```python
from build123d import *

# Parameters (mm, degrees)
BASE_FLANGE1_DEPTH      = 31.75
F_1_4_CLEARANCE_HOLE1_D = 6.7564
F_1_4_CLEARANCE_HOLE2_D = 6.7564
FILLET1_R               = 2.54


# Sheet-metal steps are written as plain solids
with BuildPart() as part:
    # Sketch1 → Base-Flange1 (new body)
    with BuildSketch(Plane(origin=(0, 0, 0), x_dir=(0, 0, -1), z_dir=(1, 0, 0))):
        with BuildLine():
            Line((-28.575, 0), (-3.9878, 0))
            ThreePointArc((-3.9878, 0), (-1.167999578, 1.167999578), (0, 3.9878))
            Line((0, 3.9878), (0, 50.8))
            Line((0, 50.8), (-1.9939, 50.8))
            Line((-1.9939, 50.8), (-1.9939, 3.9878))
            ThreePointArc((-1.9939, 3.9878), (-2.577899789, 2.577899789), (-3.9878, 1.9939))
            Line((-3.9878, 1.9939), (-28.575, 1.9939))
            Line((-28.575, 1.9939), (-28.575, 0))
        make_face()
    extrude(amount=BASE_FLANGE1_DEPTH)

    # 1/4 Clearance Hole1 (through all)
    with Locations(Plane.XY.offset(1.9939)):
        with Locations((15.875, 41.275)):
            Hole(F_1_4_CLEARANCE_HOLE1_D / 2)

    # 1/4 Clearance Hole2 (through all)
    with Locations(Plane(origin=(0, 1.9939, 0), x_dir=(1, 0, 0), z_dir=(0, 1, 0))):
        with Locations((15.875, -22.225)):
            Hole(F_1_4_CLEARANCE_HOLE2_D / 2)

    # Fillet1
    fillet1_edges = [part.edges().sort_by_distance(p)[0] for p in [
        (31.75, 0.99695, 28.575),
        (0, 0.99695, 28.575),
        (31.75, 50.8, 0.99695),
        (0, 50.8, 0.99695),
    ]]
    fillet(fillet1_edges, radius=FILLET1_R)


solid = part.part
```
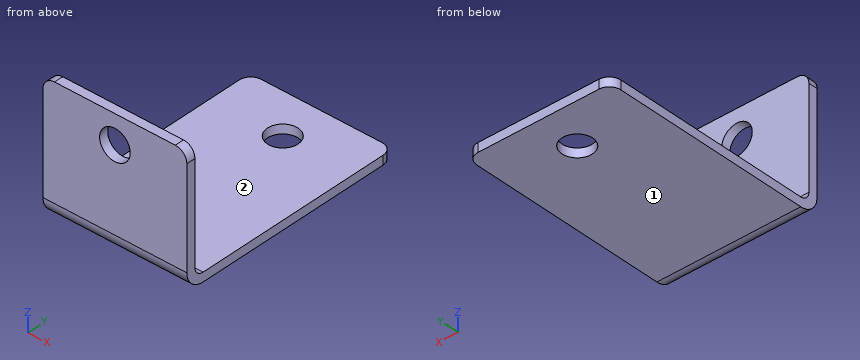
The listing builds one solid part. Answer for the finished solid, in the listing's coordinates (mm). Face numbers are marked on the shaded views. A direction names the side the tool comes from. Round coordinates to 2 decimals unless told otherwise and drop trailing zeros. Order: outer loops, then holes, each group sorted by start corner. A loop starts at its lowest first (then second) coordinate and runs counter-clockwise, first axis right, second up. Notation, with made-up numbers: (44, -6.75) -> (91, -6.75) arc R19 cw to (91, 18.25) -> close; hole circle Ø4 at (-34.5, 72.5). An arc over 180 degrees is marked (long way). Answer as CSV lines item,"result". Start each with the question number.
(1) A tool of negligible diameter and unlimited length cuts with its end or side. For the marked faces 1 and 2, from which of +Z, -Z, +X, -X, +Y, -Y can it reach the whole face along a straight path? Write none if from no direction.
(2) Flat-ended cylindrical pins translate along their axes: pin 1 Ø12.5 at (x, z) = (13, 11) entering from +Y; pin 2 Ø12 at (x, y) = (14, 42) entering from +Z. Find the tip coordinate at first contact, or state that the pin passes through.
(3) The part is cut by section D-D (y = 34). Determine the outline of the cut face in (x, z), then the cut area to 3 significant figures.
(4) Find the intervals of material crossed by probe 1 along Y at (x, z) = (17, 11.5); probe 2 along Y at (x, z) = (30.5, 2.75), in increasing order. Write a range as from..to.
(5) The part is cut by section C-C (x = 14). Determine the outline of the cut face in (y, z) (3 decimals).
(6) The part is cut by section B-B (z = 24). Determine the outline of the cut face in (x, y).
(7) The part is cut by section A-A (x = 7). Determine the outline of the cut face in (y, z) (3 decimals), then the cut area to 3 significant figures.
Evaluation:
1,face 1,"-Z, +X, -X, +Y, -Y"
1,face 2,"+Z, +X, -X, +Y"
2,pin 1,"y = 1.99"
2,pin 2,"z = 1.99"
3,outline,"(0, 0) -> (31.75, 0) -> (31.75, 1.99) -> (0, 1.99) -> close"
3,area,"63.3 mm²"
4,probe 1,"0..1.99"
4,probe 2,"0.2..2.42"
5,outline,"(0, 3.988) arc R3.988 ccw to (3.988, 0) -> (38.465, 0) -> (38.465, 1.994) -> (3.988, 1.994) arc R1.994 cw to (1.994, 3.988) -> (1.994, 19.415) -> (0, 19.415) -> close; (0, 25.035) -> (1.994, 25.035) -> (1.994, 28.575) -> (0, 28.575) -> close; (44.085, 0) -> (50.8, 0) -> (50.8, 1.994) -> (44.085, 1.994) -> close"
6,outline,"(0, 0) -> (13, 0) -> (13, 1.99) -> (0, 1.99) -> close; (18.75, 0) -> (31.75, 0) -> (31.75, 1.99) -> (18.75, 1.99) -> close"
7,outline,"(0, 3.988) arc R3.988 ccw to (3.988, 0) -> (50.8, 0) -> (50.8, 1.994) -> (3.988, 1.994) arc R1.994 cw to (1.994, 3.988) -> (1.994, 28.575) -> (0, 28.575) -> close"
7,area,"152 mm²"
